Read the model definition and answer for the solid it produces. Units are mm, in the model's axes. Give positions to 0.01 mm unless a question says otherwise; leave off trailing zeros. Order: outer loops, then holes, each group sorted by start corner. A loop starts at its lowest first (then second) coordinate and runs counter-clockwise, first axis right, second up. Notation, with made-up numbers: (-22, 74.25) - (32, 74.25) arc R11 ccw to (32, 78.25) - close; hole circle Ø5 at (-16, -18). An arc over 180 degrees is marked (long way). Use a Markdown table: item, result. Add a question column.
1. A cutting plane is placed at A-A on x = -8.8. Determine the outline of the cut face in (y, z), and give its area (3 significant figures).
2. A flat-ended cylindrical pin translates along its axis: P1, Ø2, axis at x = -8.8, z = -0.36, coming from the -Y side. Find the tip coordinate at first contact, or state that the pin passes through.
3. Consider L1, parallel to X at y = 1.05, z = -2.5 (3 decimals); L2, parallel to Z at x = -8.8, y = 0.7; L3, parallel to X at y = 0.95, z = 2.25 (3 decimals). Determine where each line is inside the solid, lowest interval first.
4. A cutting plane is placed at B-B on y = 0.3. State how many separate pieces and enclosed holes the cut face has, and give its area (3 significant figures).
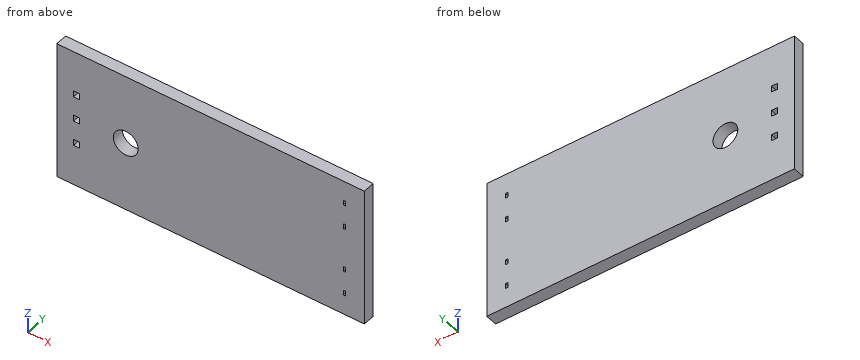
```python
from build123d import *

# Parameters (mm, degrees)
SKETCH1_W           = 31
SKETCH1_H           = 14
BOSS_EXTRUDE1_DEPTH = 1.2
SKETCH2_R           = 1.25
SKETCH2_W           = 0.63
SKETCH2_H           = 0.63
SKETCH2_W_2         = 0.25
SKETCH2_H_2         = 0.5
CUT_EXTRUDE1_DEPTH  = 2.2


with BuildPart() as part:
    # Sketch1 → Boss-Extrude1 (new body)
    with BuildSketch(Plane(origin=(0, 0, 0), x_dir=(1, 0, 0), z_dir=(0, 1, 0))):
        with Locations((-0.25, 0.35546875)):
            Rectangle(SKETCH1_W, SKETCH1_H)
    extrude(amount=BOSS_EXTRUDE1_DEPTH)

    # Sketch2 → Cut-Extrude1 (cut, through all)
    with BuildSketch(Plane(origin=(0, 1.2, 0), x_dir=(1, 0, 0), z_dir=(0, 1, 0))):
        with Locations((-8.8, 0.35546875)):
            Circle(SKETCH2_R)
        with Locations((-13.75, 2.91546875)):
            Rectangle(SKETCH2_W, SKETCH2_H)
        with Locations((-13.75, 0.35546875)):
            Rectangle(SKETCH2_W, SKETCH2_H)
        with Locations((-13.75, -2.20453125)):
            Rectangle(SKETCH2_W, SKETCH2_H)
        with Locations((13.25, -4.39453125)):
            Rectangle(SKETCH2_W_2, SKETCH2_H_2)
        with Locations((13.25, -1.89453125)):
            Rectangle(SKETCH2_W_2, SKETCH2_H_2)
        with Locations((13.25, 2.60546875)):
            Rectangle(SKETCH2_W_2, SKETCH2_H_2)
        with Locations((13.25, 5.10546875)):
            Rectangle(SKETCH2_W_2, SKETCH2_H_2)
    extrude(amount=-CUT_EXTRUDE1_DEPTH, mode=Mode.SUBTRACT)


solid = part.part
```
Output values:
| question | item | result |
|---|---|---|
| 1 | outline | (0, -7.36) - (1.2, -7.36) - (1.2, -1.61) - (0, -1.61) - close; (0, 0.89) - (1.2, 0.89) - (1.2, 6.64) - (0, 6.64) - close |
| 1 | area | 13.8 mm² |
| 2 | P1 | through |
| 3 | L1 | -15.75 to 13.125, 13.375 to 15.25 |
| 3 | L2 | -7.36 to -1.61, 0.89 to 6.64 |
| 3 | L3 | -15.75 to -14.065, -13.435 to 15.25 |
| 4 | separate pieces | 1 |
| 4 | enclosed holes | 8 |
| 4 | area | 427 mm² |
